Read the model definition and answer for the solid it produces. Units are mm, in the model's axes. Face numbers are marked on the shaded views. A direction names the side the tool comes from. Give positions to 0.01 mm unless a question says otherwise; leave off trailing zeros. Order: outer loops, then holes, each group sorted by start corner. A loop starts at its lowest first (then second) coordinate and runs counter-clockwise, first axis right, second up. Notation, with made-up numbers: M 18,20 L 57,20 A15 ccw 57,41 Z; hole C -26.5,75 d3. An arc over 180 degrees is marked long. One line per item, written item: value.
Autodesk Fusion 360 part; units mm, degrees
sketch "Sketch1" plane through (0, 0, 0) normal (0, 1, 0) x (1, 0, 0)
  line L0 (30, 30) -> (30, -30)
  line L1 (30, -30) -> (-30, -30)
  line L2 (-30, -30) -> (-30, 30)
  line L3 (-30, 30) -> (30, -30) construction
  line L4 (30, 30) -> (-30, -30) construction
  line L5 (10, 30) -> (10, 50)
  line L6 (10, 50) -> (-10, 50)
  line L7 (-10, 50) -> (-10, 30)
  line L8 (-30, 30) -> (-10, 30)
  line L9 (10, 30) -> (30, 30)
  circle A0 centre (0, 43) radius 2.6
  line L10 (-30, 0) -> (30, 0) construction
  circle A1 centre (0, 21.5) radius 2.6
  circle A2 centre (-23, 21.5) radius 2.6
  circle A3 centre (23, 21.5) radius 2.6
  circle A4 centre (-23, 0) radius 2.6
  circle A5 centre (0, 0) radius 2.6
  circle A6 centre (23, 0) radius 2.6
  circle A7 centre (-23, -21.5) radius 2.6
  circle A8 centre (23, -21.5) radius 2.6
  line L11 (-2.6, -21) -> (-2.6, -22)
  arc A9 (-2.6, -22) -> (2.6, -22) centre (0, -22) ccw
  line L12 (2.6, -22) -> (2.6, -21)
  arc A10 (2.6, -21) -> (-2.6, -21) centre (0, -21) ccw
  point P0 (0, -21.5)
  dimension "d4" = 60
  dimension "d5" = 60
  dimension "d7" = 20
  dimension "d8" = 20
  dimension "d9" = 5.2
  dimension "d10" = 7
  dimension "d11" = 5.2
  dimension "d12" = 21.5
  dimension "d13" = 5.2
  dimension "d14" = 5.2
  dimension "d15" = 23
  dimension "d16" = 23
  dimension "d28" = 5.2
  dimension "d29" = 0.5
extrude "Extrude1" add sketch "Sketch1" along normal blind 6
chamfer "Chamfer1" distance 6 angle 45 4 edges at (30, 3, 30) (30, 3, -30) (-30, 3, 30) (-30, 3, -30)
fillet "Fillet1" radius 3 2 edges at (10, 3, -50) (-10, 3, -50)
fillet "Fillet2" radius 3 2 edges at (10, 3, -30) (-10, 3, -30)
sketch "Sketch2" plane through (0, 6, 0) normal (0, 1, 0) x (-1, 0, 0)
  arc A0 (7, -50) -> (10, -47) centre (7, -47) ccw
  line L0 (10, -47) -> (10, -33)
  arc A1 (13, -30) -> (10, -33) centre (13, -33) ccw
  line L1 (13, -30) -> (24, -30)
  line L2 (24, -30) -> (30, -24)
  line L3 (30, -24) -> (30, 24)
  line L4 (30, 24) -> (24, 30)
  line L5 (24, 30) -> (-24, 30)
  line L6 (-24, 30) -> (-30, 24)
  line L7 (-30, 24) -> (-30, -24)
  line L8 (-30, -24) -> (-24, -30)
  line L9 (-24, -30) -> (-13, -30)
  arc A2 (-10, -33) -> (-13, -30) centre (-13, -33) ccw
  line L10 (-10, -33) -> (-10, -47)
  arc A3 (-10, -47) -> (-7, -50) centre (-7, -47) ccw
  line L11 (-7, -50) -> (7, -50)
  circle A4 centre (23, 0) radius 2.6
  circle A5 centre (0, 0) radius 2.6
  circle A6 centre (0, -21.5) radius 2.6
  circle A7 centre (0, -43) radius 2.6
  circle A8 centre (23, 21.5) radius 2.6
  arc A9 (-2.6, 21) -> (2.6, 21) centre (0, 21) ccw
  line L12 (-2.6, 21) -> (-2.6, 22)
  arc A10 (2.6, 22) -> (-2.6, 22) centre (0, 22) ccw
  line L13 (2.6, 22) -> (2.6, 21)
  circle A11 centre (23, -21.5) radius 2.6
  circle A12 centre (-23, 0) radius 2.6
  circle A13 centre (-23, -21.5) radius 2.6
  circle A14 centre (-23, 21.5) radius 2.6
  line L14 (10, 12) -> (-10, 12)
  line L15 (-10, 12) -> (-10, 30)
  line L16 (10, 30) -> (10, 12)
  line L17 (0, -30) -> (-9, -30)
  line L18 (0, -30) -> (9, -30)
  line L19 (9, -30) -> (9, -12)
  line L20 (-9, -30) -> (-9, -12)
  line L21 (30, -12) -> (9, -12)
  line L22 (-9, -12) -> (-30, -12)
  dimension "d40" = 20
  dimension "d41" = 18
  dimension "d44" = 10
  dimension "d45" = 9
  dimension "d46" = 9.5
  dimension "d47" = 9
  dimension "d48" = 9
  dimension "d49" = 8.5
extrude "Extrude2" cut sketch "Sketch2" against normal blind 6 contours A0 L0 A1 L1 L2 L3 L7 L8 L9 A2 L10 A3 L11 L17 L18 L19 L20 L21 L22 | L5 L14 L15 L16
sketch "Sketch3" plane through (0, 6, 0) normal (0, 1, 0) x (-1, 0, 0)
  circle A0 centre (0, 0) radius 2.6
  circle A1 centre (23, 21.5) radius 2.6
  circle A2 centre (0, -21.5) radius 2.6
  circle A3 centre (23, 0) radius 2.6
  circle A4 centre (-23, 0) radius 2.6
  circle A5 centre (-23, 21.5) radius 2.6
  line L0 (10, 30) -> (10, 12)
  line L1 (10, 12) -> (-10, 12)
  line L2 (-10, 12) -> (-10, 30)
  line L3 (-10, 30) -> (-24, 30)
  line L4 (-24, 30) -> (-30, 24)
  line L5 (-30, 24) -> (-30, -12)
  line L6 (-30, -12) -> (-9, -12)
  line L7 (-9, -12) -> (-9, -30)
  line L8 (-9, -30) -> (9, -30)
  line L9 (9, -30) -> (9, -12)
  line L10 (9, -12) -> (30, -12)
  line L11 (30, -12) -> (30, 24)
  line L12 (30, 24) -> (24, 30)
  line L13 (24, 30) -> (10, 30)
  circle A6 centre (15, 12) radius 1.5
  circle A7 centre (-15, 12) radius 1.5
  circle A8 centre (6, -11.9995) radius 1.5
  circle A9 centre (-6, -11.9995) radius 1.5
  dimension "d53" = 3
  dimension "d54" = 15
  dimension "d55" = 12
  dimension "d56" = 3
  dimension "d57" = 15
  dimension "d58" = 12
  dimension "d59" = 3
  dimension "d60" = 3
  dimension "d61" = 6
  dimension "d62" = 6
  dimension "d63" = 13.416
  dimension "d64" = 13.416
extrude "Extrude3" cut sketch "Sketch3" against normal blind 6 contours A6 | A7 | A8 | A9
equation "larger_hole_radii = 2.6 mm"
equation "small_hole_Radii = 1.25 mm"
equation "base_sqaure_dim = 60 mm"
equation "d4 = base_sqaure_dim"
equation "d5 = base_sqaure_dim"
equation "square_extension = 20 mm"
equation "d7 = square_extension"
equation "d8 = square_extension"
equation "d9 = larger_hole_radii * 2"
equation "d11 = larger_hole_radii * 2"
equation "d13 = 2 * larger_hole_radii"
equation "d14 = 2 * larger_hole_radii"
equation "dist_between_Rows = 21.50 mm"
equation "slot_height = 5.20 mm"
equation "slot_width = 0.50 mm"
equation "d28 = slot_height"
equation "d29 = slot_width"
equation "ext = 6.0 mm"
equation "d31 = ext"
equation "d33 = ext"
equation "fillet_top = 3 mm"
equation "d36 = fillet_top"
equation "d38 = fillet_top"
equation "slot_square_cutout_height = 18 mm"
equation "d40 = square_extension"
equation "d41 = slot_square_cutout_height"
equation "d44 = square_extension / 2"
equation "d45 = slot_square_cutout_height / 2"
equation "d46 = square_extension / 2 - 0.50 mm"
equation "d47 = slot_square_cutout_height / 2"
equation "d48 = slot_square_cutout_height / 2"
equation "d49 = slot_square_cutout_height / 2 - 0.50 mm"
equation "new_small_hole_dia = 3 mm"
equation "d53 = new_small_hole_dia"
equation "d56 = new_small_hole_dia"
equation "d59 = new_small_hole_dia"
equation "d60 = new_small_hole_dia"
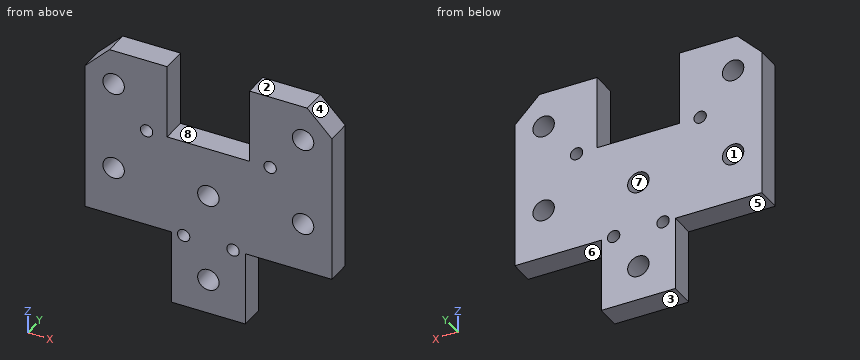
1) Determine the mould class of the marked faces 1, 2 and 3 for opening direction Z: +Z half, -Z half, draft (parallel to the pull), parting line (faces both ways), or undercut.
Reported:
face 1: undercut
face 2: +Z half
face 3: -Z half
2) Find section A-A, the plane z = -21.5. Write down the section's boundary in (x, y), plus the area to 3 significant figures.
Reported:
outline: M -9,0 L -2.6,0 L -2.6,6 L -9,6 Z; M 2.6,0 L 9,0 L 9,6 L 2.6,6 Z
area: 76.8 mm^2
3) Consider probe 1 along X at (y, z) = (5.05, 0); probe 2 along Z at (x, y) = (-23, 1.7); probe 3 along Z at (x, y) = (0, 4.75). Determine where each line is inside the solid, lowest interval first.
Reported:
probe 1: x = -30 to -25.6, -20.4 to -2.6, 2.6 to 20.4, 25.6 to 30
probe 2: z = -12 to -2.6, 2.6 to 18.9, 24.1 to 30
probe 3: z = -30 to -24.1, -18.9 to -2.6, 2.6 to 12
4) Each of these flat-tipped pins is pushed along its axis until it touches: pin 1 Ø4 at (x, z) = (-23, 0) entering from -Y; pin 2 Ø1.8 at (x, y) = (-16, 2) entering from -Z; pin 3 Ø3 at (y, z) = (4.5, -24.5) entering from +X. Where does it stop, or does it pass through?
Reported:
pin 1: passes through
pin 2: stops at z = -12
pin 3: stops at x = 9
5) Find section C-C, the plane z = 20. Write down the section's boundary in (x, y).
Reported:
outline: M -30,0 L -25.12,0 L -25.12,6 L -30,6 Z; M -20.88,0 L -10,0 L -10,6 L -20.88,6 Z; M 10,0 L 20.88,0 L 20.88,6 L 10,6 Z; M 25.12,0 L 30,0 L 30,6 L 25.12,6 Z
6) Which of the six approach directions +Z, -Z, +X, -X, +Y, -Y give full straight-line access (tool end or side, diameter ignored) to the marked faces 4, 5, 6, 7 and 8?
Reported:
face 4: +Z, +X, +Y, -Y
face 5: -Z, -X, +Y, -Y
face 6: -Z, +X, +Y, -Y
face 7: +Y, -Y
face 8: +Z, +Y, -Y
7) Find section B-B, the plane x = -15. Write down the section's boundary in (y, z).
Reported:
outline: M 0,-12 L 6,-12 L 6,10.5 L 0,10.5 Z; M 0,13.5 L 6,13.5 L 6,30 L 0,30 Z
8) Find section D-D, the plane x = -23. Write down the section's boundary in (y, z).
Reported:
outline: M 0,-12 L 6,-12 L 6,-2.6 L 0,-2.6 Z; M 0,2.6 L 6,2.6 L 6,18.9 L 0,18.9 Z; M 0,24.1 L 6,24.1 L 6,30 L 0,30 Z
